Check sheet for the modelled part. Datum: model origin and axes. Units: mm. Face numbers are marked on the shaded views. A direction names the side the tool comes from. Coordinates: 2 decimals unless noted, no trailing zeros. Write each loop counter-clockwise with the first axis right and the second up, starting at its lowest first coordinate (ties: lowest second). Pieces come first, ordered by that corner, then holes. Notation, with made-up numbers: (39.25, 75.5) -> (91.25, 75.5) arc R20 ccw to (91.25, 96.5) -> close; hole circle Ø3 at (9.25, 88). An arc over 180 degrees is marked (long way). One line per item, written item: value. Start each with the question number.
1) Gauge pin test, flat ends, axial feed: P1, Ø12, axis at y = 21, z = -6, coming from the +X side; P2, Ø10, axis at x = -10, z = -28, coming from the -Y side; P3, Ø8, axis at x = -2.5, z = -24.5, coming from the +Y side; P4, Ø3, axis at x = 2.5, y = 22, coming from the +Z side. Record the tip position at first contact, or that the pin passes through.
2) Draft check along Z on the marked faces 3, 4, 5 and 6. Enter one of: +Z half, -Z half, draft (parallel to the pull), parting line (faces both ways), or undercut.
3) Sectioned sample at B-B on y = 3.25. Enter the section's corners in (x, z), plus the area to 3 significant figures.
4) Scan lines: line 1 along Y through (x, z) = (-0.5, -20); line 2 along Y through (x, z) = (6, -27); line 3 along Y through (x, z) = (0.5, -6.5). Record each from-to range of solid material in increasing order. Write a range as [from, to].
5) Sectioned sample at A-A on y = 12.25. Enter the section's corners in (x, z).
6) Sectioned sample at D-D on x = -25. Enter the section's corners in (y, z).
7) Set-up check for the marked faces 1 and 2: record each of +Z, -Z, +X, -X, +Y, -Y from which the full face is reachable in a straight line by a thin tool's end or side.
8) Sectioned sample at C-C on z = -22. Give the number of separate pieces and of enclosed holes in the cut face, plus the area to 3 significant figures.
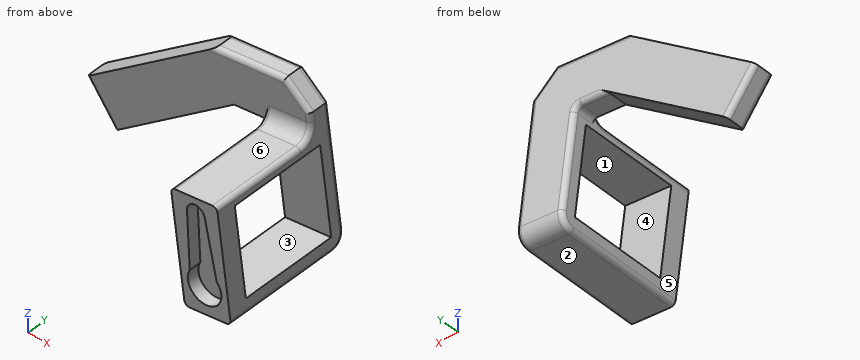
```python
from build123d import *

# Parameters (mm, degrees)
EXTRUDE_THIN1_DEPTH = 27.5
CUT_EXTRUDE1_DEPTH  = 23
CUT_EXTRUDE2_DEPTH  = 2.55
FILLET1_R           = 3
FILLET2_R           = 1
CUT_EXTRUDE3_REACH  = 66.468
SKETCH5_W           = 18.148983488
SKETCH5_H           = 20.5


# Read off the part's stored shape, not the designer's step: Extrude-Thin1
with BuildPart() as part:
    # Extrude-Thin1 outline → Extrude-Thin1 (new body)
    with BuildSketch(Plane(origin=(0, 0, 0), x_dir=(1, 0, 0), z_dir=(0, 1, 0))):
        Polygon((-10.904976106, 11.527203276), (-36.538248885, 31.213507371), (-42.629212569, 23.282545173), (-14.870844874, 1.964172277), (0, 0), (5.378547824, 4.483293206), (9.045002742, 32.242203638), (-0.868893841, 33.551651823), (-3.900133282, 10.601988993), align=None)
    extrude(amount=EXTRUDE_THIN1_DEPTH)

    # Sketch2 → Cut-Extrude1 (cut)
    with BuildSketch(Plane.XZ):
        Polygon((-3.900133282, -10.601988993), (6.0137633, -9.292540808), (4.704315116, 0.621355774), (-14.870844874, -1.964172277), (-42.629212569, -23.282545173), (-36.538248885, -31.213507371), (-10.904976106, -11.527203276), align=None)
    extrude(amount=-CUT_EXTRUDE1_DEPTH, mode=Mode.SUBTRACT)

    # Sketch3 → Cut-Extrude2 (cut)
    with BuildSketch(Plane.XZ):
        with BuildLine():
            Line((3.380947821, -12.850204555), (5.968175927, -24.824313447))
            ThreePointArc((5.968175927, -24.824313447), (3.826164813, -30.914148414), (0.176477543, -25.589293076))
            Line((0.176477543, -25.589293076), (-0.433912303, -13.354079255))
            ThreePointArc((-0.433912303, -13.354079255), (1.241314096, -11.34411656), (3.380947821, -12.850204555))
        make_face()
    extrude(amount=-CUT_EXTRUDE2_DEPTH, mode=Mode.SUBTRACT)

    # Fillet1
    fillet1_edges = [part.edges().sort_by_distance(p)[0] for p in [
        (4.08805445, 27.5, -32.89692773),
        (1.056815009, 23, -9.947264901),
    ]]
    fillet(fillet1_edges, radius=FILLET1_R)

    # Fillet2
    fillet2_edges = [part.edges().sort_by_distance(p)[0] for p in [
        (-3.900133282, 25.25, -10.601988993),
        (-7.435422437, 27.5, -0.982086139),
        (2.689273912, 27.5, -2.241646603),
        (-3.900133282, 10, -10.601988993),
        (-39.583730727, 23, -27.248026272),
        (-7.435422437, 23, -0.982086139),
        (-7.402554694, 27.5, -11.064596135),
        (2.689273912, 23, -2.241646603),
        (-0.868893841, 12.25, -33.551651823),
        (9.045002742, 12.25, -32.242203638),
        (6.0137633, 10, -9.292540808),
        (7.015358055, 27.5, -16.875663935),
        (5.499738334, 23, -5.40083252),
        (8.929944194, 26.621320344, -31.371089714),
        (-2.580930789, 27.5, -20.589735921),
        (-0.983952389, 26.621320344, -32.680537899),
        (5.898704753, 22.121320344, -8.421426884),
        (-4.01519183, 22.121320344, -9.730875069),
        (-39.583730727, 27.5, -27.248026272),
    ]]
    fillet(fillet2_edges, radius=FILLET2_R)

    # Sketch5 → Cut-Extrude3 (cut, up to next)
    with BuildSketch(Plane(origin=(4.704315116, 0, 0.621355774), x_dir=(0.13094481849155867, 0, -0.9913896582626898), z_dir=(0.9913896582626898, 0, 0.13094481849155867)), mode=Mode.PRIVATE) as cut_extrude3_sk1:
        with Locations((21.074491744, 14.25)):
            Rectangle(SKETCH5_W, SKETCH5_H)
    cut_extrude3_tool1 = extrude(cut_extrude3_sk1.sketch, amount=-CUT_EXTRUDE3_REACH, mode=Mode.PRIVATE) & part.part
    add(cut_extrude3_tool1.solids().sort_by_distance((7.463911, 14.25, -20.271677))[0], mode=Mode.SUBTRACT)


solid = part.part
```
Answers:
1. P1: stops at x = 6.28
1. P2: passes through
1. P3: stops at y = 27.5
1. P4: stops at z = -1.83
2. face 3: undercut
2. face 4: undercut
2. face 5: -Z half
2. face 6: +Z half
3. outline: (-3.77, -11.59) -> (-1, -32.56) arc R1 ccw to (0.12, -33.42) -> (8.05, -32.37) arc R1 ccw to (8.91, -31.25) -> (6.14, -10.28) arc R1 ccw to (5.02, -9.42) -> (-2.91, -10.47) arc R1 ccw to start
3. area: 231 mm2
4. line 1: y = [0, 4], [24.5, 27.5]
4. line 2: y = [2.55, 4], [24.5, 27.5]
4. line 3: y = [23, 27.5]
5. outline: (-3.77, -11.59) -> (-3.64, -12.58) -> (6.28, -11.28) -> (6.14, -10.28) arc R1 ccw to (5.02, -9.42) -> (-2.91, -10.47) arc R1 ccw to start; (-1.26, -30.58) -> (-1, -32.56) arc R1 ccw to (0.12, -33.42) -> (8.05, -32.37) arc R1 ccw to (8.91, -31.25) -> (8.65, -29.27) -> close
6. outline: (23, -22.35) -> (27.5, -22.35) -> (27.5, -9.74) -> (23, -9.74) -> close
7. face 1: +X
7. face 2: -Z, +X, +Y, -Y
8. separate pieces: 3
8. enclosed holes: 0
8. area: 130 mm2
